Can you work these out from the drawing? Everything is in mm from the part's minimum corner. Give positions to 0.01 mm unless a question says otherwise; leave off trailing zeros. Order: outer loops, then holes, each group sorted by start corner. A loop starts at its lowest first (then second) coordinate and runs counter-clockwise, first axis right, second up. Notation, with made-up numbers: M 74,87 L 129,87 A11 cw 129,102 Z; hole C 24,72 d10. An arc over 180 degrees is marked long. Use a Markdown table: item, result. Add a question column.
Item 1: I'm going to push flat-ended pins straight in: pin 1 Ø1 at (x, z) = (1.5, 1.5) entering from -Y; pin 2 Ø1.5 at (x, z) = (13.5, 2) entering from -Y. Where does each tip first touch, or does it pass through?
Item 2: Suppose I cut it at A-A on z = 1.5. Write out the boundary of the cut face in (x, y), plus the area to 3 significant figures.
Item 3: Suppose I cut it at C-C on y = 3.4. Write out the boundary of the cut face in (x, z).
Item 4: If I drill on L1, parallel to Y at x = 36.75, z = 0.65; L2, parallel to X at y = 1.3, z = 1.5; L3, parallel to X at y = 1.75, z = 1.5, over which ranges is the centre line in solid material (lowest first)? Write a range as from..to.
Item 5: Suppose I cut it at B-B on x = 1.5. Write out the boundary of the cut face in (y, z), plus the area to 3 significant figures.
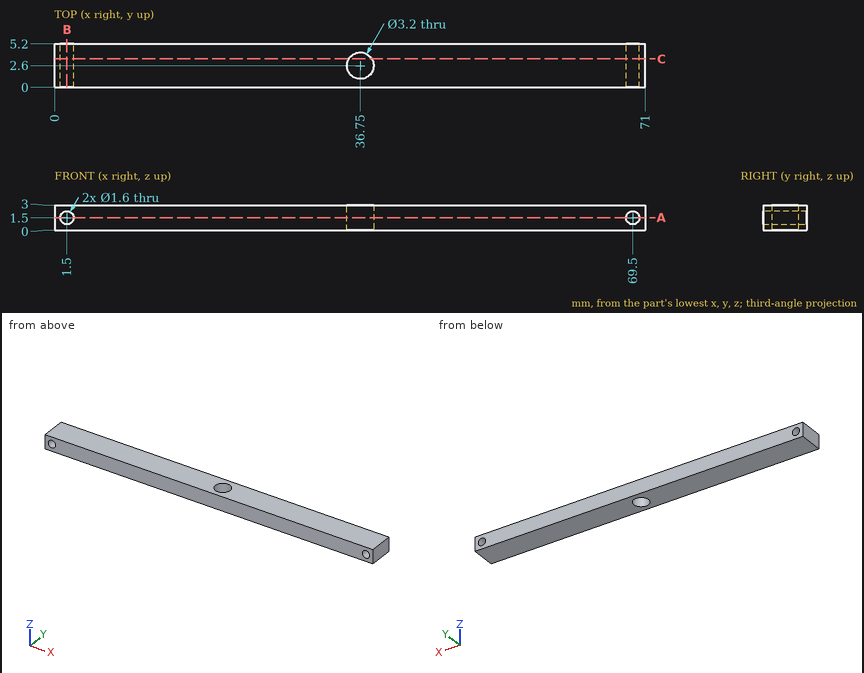
Findings below:
| question | item | result |
|---|---|---|
| 1 | pin 1 | passes through |
| 1 | pin 2 | stops at y = 0 |
| 2 | outline | M 0,0 L 0.7,0 L 0.7,5.2 L 0,5.2 Z; M 2.3,0 L 68.7,0 L 68.7,5.2 L 2.3,5.2 Z; M 70.3,0 L 71,0 L 71,5.2 L 70.3,5.2 Z; hole C 36.75,2.6 d3.2 |
| 2 | area | 345 mm^2 |
| 3 | outline | M 0,0 L 35.36,0 L 35.36,3 L 0,3 Z; M 38.14,0 L 71,0 L 71,3 L 38.14,3 Z; hole C 1.5,1.5 d1.6; hole C 69.5,1.5 d1.6 |
| 4 | L1 | y = 0..1, 4.2..5.2 |
| 4 | L2 | x = 0..0.7, 2.3..35.82, 37.68..68.7, 70.3..71 |
| 4 | L3 | x = 0..0.7, 2.3..35.39, 38.11..68.7, 70.3..71 |
| 5 | outline | M 0,0 L 5.2,0 L 5.2,0.7 L 0,0.7 Z; M 0,2.3 L 5.2,2.3 L 5.2,3 L 0,3 Z |
| 5 | area | 7.28 mm^2 |
